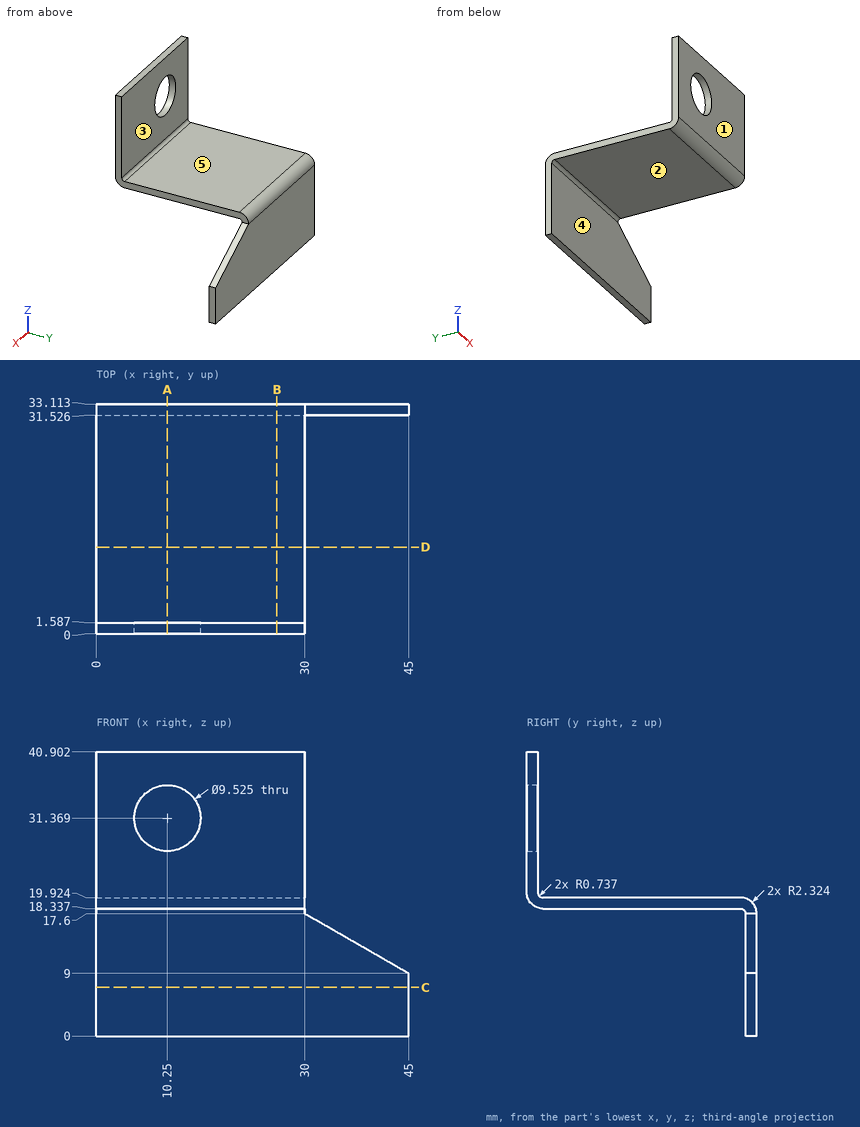
Print and shaded views of the part. All mm, measured from the part's lowest x, y and z. A direction names the side the tool comes from. Round coordinates to 2 decimals unless told otherwise and drop trailing zeros. Write each loop counter-clockwise with the first axis right and the second up, starting at its lowest first coordinate (ties: lowest second). Pieces come first, ordered by that corner, then holes.
(1) Slice it at C-C, the plane z = 7. Write the cut outline in (x, y) (1 decimal).
(2) Slice it at B-B, the plane x = 26. Write the cut outline in (y, z) (1 decimal).
(3) 3-axis set-ups, long thin cutter, end or side, ignore diameter. For the marked faces 1 and 2: which of +Z, -Z, +X, -X, +Y, -Y reach the whole face in a straight line?
(4) Slice it at A-A, the plane x = 10.25. Write the cut outline in (y, z) (1 decimal).
(5) Probe line 1 along Z through (x, y) = (24, 19) (1 decimal); line 2 along Y through (x, z) = (29.5, 27); line 3 along Y through (x, z) = (34.5, 8.5) (1 decimal). List the from-to ranges inside material, lowest first.
(6) Mould opens along Y. For the marked faces 3, 4 and 5 say: pulls with the +Y half, pulls with the -Y half, needs draft (parallel to the pull), parting line crosses it, or undercut.
(7) Drop flat-ended pins along their axis: P1, Ø6, axis at x = 24.5, z = 35, coming from the +Y side; P2, Ø4, axis at x = 13, y = 28, coming from the +Z side; P3, Ø2, axis at x = 19, z = 29, coming from the -Y side; P4, Ø19.5, axis at x = 26.5, z = 5, coming from the -Y side. Give the stop position or say it passes through.
(8) Slice it at D-D, the plane y = 12.5. Write the cut outline in (x, z) (1 decimal).
From the geometry:
1. outline: (0, 31.5) - (45, 31.5) - (45, 33.1) - (0, 33.1) - close
2. outline: (0, 20.7) arc R2.3 ccw to (2.3, 18.3) - (30.8, 18.3) arc R0.7 cw to (31.5, 17.6) - (31.5, 0) - (33.1, 0) - (33.1, 17.6) arc R2.3 ccw to (30.8, 19.9) - (2.3, 19.9) arc R0.7 cw to (1.6, 20.7) - (1.6, 40.9) - (0, 40.9) - close
3. face 1: +Z, -Z, +X, -X, -Y
3. face 2: -Z, +X, -X, -Y
4. outline: (0, 20.7) arc R2.3 ccw to (2.3, 18.3) - (30.8, 18.3) arc R0.7 cw to (31.5, 17.6) - (31.5, 0) - (33.1, 0) - (33.1, 17.6) arc R2.3 ccw to (30.8, 19.9) - (2.3, 19.9) arc R0.7 cw to (1.6, 20.7) - (1.6, 26.6) - (0, 26.6) - close; (0, 36.1) - (1.6, 36.1) - (1.6, 40.9) - (0, 40.9) - close
5. line 1: z = 18.3 to 19.9
5. line 2: y = 0 to 1.59
5. line 3: y = 31.5 to 33.1
6. face 3: pulls with the +Y half
6. face 4: pulls with the -Y half
6. face 5: needs draft
7. P1: stops at y = 1.59
7. P2: stops at z = 19.92
7. P3: stops at y = 0
7. P4: stops at y = 31.53
8. outline: (0, 18.3) - (30, 18.3) - (30, 19.9) - (0, 19.9) - close
